Read the model definition and answer for the solid it produces. Units are mm, in the model's axes. Round coordinates to 2 decimals unless told otherwise and drop trailing zeros. Order: outer loops, then holes, each group sorted by start corner. A loop starts at its lowest first (then second) coordinate and runs counter-clockwise, first axis right, second up.
from build123d import *

# Parameters (mm, degrees)
SKETCH1_W           = 250
SKETCH1_H           = 340.4
SKETCH1_R           = 2.1
SKETCH1_R_2         = 2.5
SKETCH1_R_3         = 1.59
SKETCH1_R_4         = 11.75
SKETCH1_W_2         = 33
SKETCH1_H_2         = 90
BOSS_EXTRUDE1_DEPTH = 5
SKETCH12_W          = 250
SKETCH12_H          = 5
CUT_EXTRUDE2_DEPTH  = 83
CUT_EXTRUDE3_DEPTH  = 6
SKETCH15_W          = 30.082256647
SKETCH15_H          = 10
SKETCH15_W_2        = 26.03414052
CUT_EXTRUDE4_DEPTH  = 10
SKETCH17_W          = 52.148371748
SKETCH17_H          = 66.780027045
CUT_EXTRUDE5_DEPTH  = 10


with BuildPart() as part:
    # Sketch1 → Boss-Extrude1 (new body)
    with BuildSketch(Plane.XY):
        with Locations((125, -170.2)):
            Rectangle(SKETCH1_W, SKETCH1_H)
        with Locations((125, -44.64)):
            Circle(SKETCH1_R, mode=Mode.SUBTRACT)
        with Locations((125, -4)):
            Circle(SKETCH1_R, mode=Mode.SUBTRACT)
        with Locations((246, -99.4)):
            Circle(SKETCH1_R_2, mode=Mode.SUBTRACT)
        with Locations((246, -150.4)):
            Circle(SKETCH1_R_2, mode=Mode.SUBTRACT)
        with Locations((180.06, -109.275)):
            Circle(SKETCH1_R_3, mode=Mode.SUBTRACT)
        with Locations((180.06, -140.525)):
            Circle(SKETCH1_R_3, mode=Mode.SUBTRACT)
        with Locations((125, -24.14)):
            Circle(SKETCH1_R_4, mode=Mode.SUBTRACT)
        with Locations((141.96, -109.275)):
            Circle(SKETCH1_R_3, mode=Mode.SUBTRACT)
        with Locations((154.66, -109.275)):
            Circle(SKETCH1_R_3, mode=Mode.SUBTRACT)
        with Locations((167.36, -109.275)):
            Circle(SKETCH1_R_3, mode=Mode.SUBTRACT)
        with Locations((141.96, -140.525)):
            Circle(SKETCH1_R_3, mode=Mode.SUBTRACT)
        with Locations((154.66, -140.525)):
            Circle(SKETCH1_R_3, mode=Mode.SUBTRACT)
        with Locations((167.36, -140.525)):
            Circle(SKETCH1_R_3, mode=Mode.SUBTRACT)
        with Locations((82.64, -140.525)):
            Circle(SKETCH1_R_3, mode=Mode.SUBTRACT)
        with Locations((95.34, -140.525)):
            Circle(SKETCH1_R_3, mode=Mode.SUBTRACT)
        with Locations((108.04, -140.525)):
            Circle(SKETCH1_R_3, mode=Mode.SUBTRACT)
        with Locations((82.64, -109.275)):
            Circle(SKETCH1_R_3, mode=Mode.SUBTRACT)
        with Locations((95.34, -109.275)):
            Circle(SKETCH1_R_3, mode=Mode.SUBTRACT)
        with Locations((108.04, -109.275)):
            Circle(SKETCH1_R_3, mode=Mode.SUBTRACT)
        with Locations((69.94, -140.525)):
            Circle(SKETCH1_R_3, mode=Mode.SUBTRACT)
        with Locations((69.94, -109.275)):
            Circle(SKETCH1_R_3, mode=Mode.SUBTRACT)
        with Locations((4, -150.4)):
            Circle(SKETCH1_R_2, mode=Mode.SUBTRACT)
        with Locations((4, -99.4)):
            Circle(SKETCH1_R_2, mode=Mode.SUBTRACT)
        with Locations((202.56, -124.9)):
            Rectangle(SKETCH1_W_2, SKETCH1_H_2, mode=Mode.SUBTRACT)
        with BuildLine():
            Line((146.7225, -109.275), (146.7225, -128.954634918))
            ThreePointArc((146.7225, -128.954634918), (148.31, -129.040223925), (149.8975, -128.954634918))
            Line((149.8975, -128.954634918), (149.8975, -109.275))
            ThreePointArc((149.8975, -109.275), (148.31, -107.6875), (146.7225, -109.275))
        make_face(mode=Mode.SUBTRACT)
        with BuildLine():
            Line((159.42, -109.275), (159.42, -128.954634918))
            ThreePointArc((159.42, -128.954634918), (161.01, -129.040492925), (162.6, -128.954634918))
            Line((162.6, -128.954634918), (162.6, -109.275))
            ThreePointArc((162.6, -109.275), (161.01, -107.685), (159.42, -109.275))
        make_face(mode=Mode.SUBTRACT)
        with BuildLine():
            Line((172.12, -109.275), (172.12, -128.954634918))
            ThreePointArc((172.12, -128.954634918), (173.71, -129.040492925), (175.3, -128.954634918))
            Line((175.3, -128.954634918), (175.3, -109.275))
            ThreePointArc((175.3, -109.275), (173.71, -107.685), (172.12, -109.275))
        make_face(mode=Mode.SUBTRACT)
        with BuildLine():
            Line((146.7225, -140.525), (146.7225, -160.204634918))
            ThreePointArc((146.7225, -160.204634918), (148.31, -160.290223925), (149.8975, -160.204634918))
            Line((149.8975, -160.204634918), (149.8975, -140.525))
            ThreePointArc((149.8975, -140.525), (148.31, -138.9375), (146.7225, -140.525))
        make_face(mode=Mode.SUBTRACT)
        with BuildLine():
            Line((159.42, -140.525), (159.42, -160.204634918))
            ThreePointArc((159.42, -160.204634918), (161.01, -160.290492925), (162.6, -160.204634918))
            Line((162.6, -160.204634918), (162.6, -140.525))
            ThreePointArc((162.6, -140.525), (161.01, -138.935), (159.42, -140.525))
        make_face(mode=Mode.SUBTRACT)
        with BuildLine():
            Line((172.12, -140.525), (172.12, -160.204634918))
            ThreePointArc((172.12, -160.204634918), (173.71, -160.290492925), (175.3, -160.204634918))
            Line((175.3, -160.204634918), (175.3, -140.525))
            ThreePointArc((175.3, -140.525), (173.71, -138.935), (172.12, -140.525))
        make_face(mode=Mode.SUBTRACT)
        with BuildLine():
            Line((103.2775, -109.275), (103.2775, -128.954634918))
            ThreePointArc((103.2775, -128.954634918), (101.69, -130.542134918), (100.1025, -128.954634918))
            Line((100.1025, -128.954634918), (100.1025, -109.275))
            ThreePointArc((100.1025, -109.275), (101.69, -107.6875), (103.2775, -109.275))
        make_face(mode=Mode.SUBTRACT)
        with BuildLine():
            Line((90.58, -109.275), (90.58, -128.954634918))
            ThreePointArc((90.58, -128.954634918), (88.99, -130.544634918), (87.4, -128.954634918))
            Line((87.4, -128.954634918), (87.4, -109.275))
            ThreePointArc((87.4, -109.275), (88.99, -107.685), (90.58, -109.275))
        make_face(mode=Mode.SUBTRACT)
        with BuildLine():
            Line((77.88, -109.275), (77.88, -128.954634918))
            ThreePointArc((77.88, -128.954634918), (76.29, -130.544634918), (74.7, -128.954634918))
            Line((74.7, -128.954634918), (74.7, -109.275))
            ThreePointArc((74.7, -109.275), (76.29, -107.685), (77.88, -109.275))
        make_face(mode=Mode.SUBTRACT)
        with BuildLine():
            Line((103.2775, -140.525), (103.2775, -160.204634918))
            ThreePointArc((103.2775, -160.204634918), (101.69, -161.792134918), (100.1025, -160.204634918))
            Line((100.1025, -160.204634918), (100.1025, -140.525))
            ThreePointArc((100.1025, -140.525), (101.69, -138.9375), (103.2775, -140.525))
        make_face(mode=Mode.SUBTRACT)
        with BuildLine():
            Line((90.58, -140.525), (90.58, -160.204634918))
            ThreePointArc((90.58, -160.204634918), (88.99, -161.794634918), (87.4, -160.204634918))
            Line((87.4, -160.204634918), (87.4, -140.525))
            ThreePointArc((87.4, -140.525), (88.99, -138.935), (90.58, -140.525))
        make_face(mode=Mode.SUBTRACT)
        with BuildLine():
            Line((77.88, -140.525), (77.88, -160.204634918))
            ThreePointArc((77.88, -160.204634918), (76.29, -161.794634918), (74.7, -160.204634918))
            Line((74.7, -160.204634918), (74.7, -140.525))
            ThreePointArc((74.7, -140.525), (76.29, -138.935), (77.88, -140.525))
        make_face(mode=Mode.SUBTRACT)
        with Locations((47.44, -124.9)):
            Rectangle(SKETCH1_W_2, SKETCH1_H_2, mode=Mode.SUBTRACT)
    extrude(amount=BOSS_EXTRUDE1_DEPTH)

    # Sketch12 → Cut-Extrude2 (cut)
    with BuildSketch(Plane.XZ.offset(340.4)):
        with Locations((125, 2.5)):
            Rectangle(SKETCH12_W, SKETCH12_H)
    extrude(amount=-CUT_EXTRUDE2_DEPTH, mode=Mode.SUBTRACT)

    # Sketch13 → Cut-Extrude3 (cut, through all)
    with BuildSketch(Plane.XY.offset(5)):
        with BuildLine():
            Line((48.038172449, -72.5), (25.94, -72.5))
            Line((25.94, -72.5), (25.94, -94.4))
            Line((25.94, -94.4), (0, -94.4))
            Line((0, -94.4), (0, 0))
            Line((0, 0), (109.732985845, 0))
            ThreePointArc((109.732985845, 0), (95.636754361, -50.504629365), (48.038172449, -72.5))
        make_face()
        with BuildLine():
            Line((250, 0), (250, -94.4))
            Line((250, -94.4), (224.06, -94.4))
            Line((224.06, -94.4), (224.06, -72.5))
            Line((224.06, -72.5), (201.961827551, -72.5))
            ThreePointArc((201.961827551, -72.5), (154.363245639, -50.504629365), (140.267014155, 0))
            Line((140.267014155, 0), (250, 0))
        make_face()
        with BuildLine():
            Line((62.5, -233.498107088), (62.5, -350.4))
            Line((62.5, -350.4), (187.5, -350.4))
            Line((187.5, -350.4), (187.5, -233.498107088))
            ThreePointArc((187.5, -233.498107088), (125, -170.998107088), (62.5, -233.498107088))
        make_face()
    extrude(amount=-CUT_EXTRUDE3_DEPTH, mode=Mode.SUBTRACT)

    # Sketch15 → Cut-Extrude4 (cut)
    with BuildSketch(Plane.XY.offset(5)):
        with Locations((95.497044125, -5)):
            Rectangle(SKETCH15_W, SKETCH15_H)
        with Locations((152.478897811, -5)):
            Rectangle(SKETCH15_W_2, SKETCH15_H)
    extrude(amount=-CUT_EXTRUDE4_DEPTH, mode=Mode.SUBTRACT)

    # Sketch17 → Cut-Extrude5 (cut)
    with BuildSketch(Plane.XY.offset(5)):
        with Locations((223.925814126, -225.511530956)):
            Rectangle(SKETCH17_W, SKETCH17_H)
        with Locations((26.074185874, -225.511530956)):
            Rectangle(SKETCH17_W, SKETCH17_H)
    extrude(amount=-CUT_EXTRUDE5_DEPTH, mode=Mode.SUBTRACT)


solid = part.part
Q1. For a pull along X with two mould halves and no side action, classify faces 1 (the face through (126.374, -171.013, 2.535)), 2 (the face through (92.716, -53.706, 2.535)), 3 (the face through (123, -127, 0)), 4 (the face through (136.207, -20.611, 2.465)) as released by +X, released by -X, zero draft, split by the parting line, or undercut.
Outcome:
face 1: undercut
face 2: released by -X
face 3: zero draft
face 4: undercut
Q2. Flat-ended cylindrical pins translate along their axes: pin 1 (3 mm diameter, centred on y = -198, z = 1.5, fed in from +X); pin 2 (3 mm diameter, centred on x = 140.5, z = 3.5, fed in from -Y); pin 3 (2.5 mm diameter, centred on y = -5.5, z = 3.5, fed in from -X). Find the tip coordinate at first contact, or state that the pin passes through.
Outcome:
pin 1: stops at x = 197.85
pin 2: stops at y = -173.35
pin 3: stops at x = 110.54
Q3. Straight lines are drawn through the part: probe 1 along Y at (x, z) = (246, 1.15); probe 2 along X at (y, z) = (-132, 1.4); probe 3 along Y at (x, z) = (48, 4.6). For each, find the intervals that lie inside material, in ascending order.
Outcome:
probe 1: y = -192.12 to -152.9, -147.9 to -101.9, -96.9 to -94.4
probe 2: x = 0 to 30.94, 63.94 to 186.06, 219.06 to 250
probe 3: y = -192.12 to -169.9, -79.9 to -72.5
Q4. A cutting plane is placed at A-A, the plane y = -227.5. Give the vertices of the cut face in (x, z), plus the area to 3 significant figures.
Outcome:
outline: (52.15, 0) - (62.79, 0) - (62.79, 5) - (52.15, 5) - close; (187.21, 0) - (197.85, 0) - (197.85, 5) - (187.21, 5) - close
area: 106 mm2
Q5. A cutting plane is placed at B-B, the plane y = -156. Give the number of separate pieces and of enclosed holes in the cut face, plus the area to 3 significant figures.
Outcome:
separate pieces: 9
enclosed holes: 0
area: 825 mm2
Q6. A cutting plane is placed at C-C, the plane x = 15.5. Give the vertices of the cut face in (y, z).
Outcome:
outline: (-192.12, 0) - (-94.4, 0) - (-94.4, 5) - (-192.12, 5) - close
